```python
from build123d import *

# Parameters (mm, degrees)
F0_W          = 279.4
F0_H          = 279.4
F0_R          = 12.7
F1_DEPTH      = 76.2
F0_W_2        = 304.8
F0_H_2        = 304.8
F2_DEPTH      = 101.6
F2_DEPTH_BACK = 88.9
F3_R          = 50.8
F4_W          = 241.3
F4_H          = 241.3
F5_DEPTH      = 139.7
F6_DEPTH      = 101.6


with BuildPart() as f1:
    # F0 (on Top) → F1 (new body, symmetric)
    with BuildSketch(Plane.XY):
        Rectangle(F0_W, F0_H)
        Circle(F0_R, mode=Mode.SUBTRACT)
    extrude(amount=F1_DEPTH, both=True)

    # F0 (on Top) → F2 (join, two sides)
    with BuildSketch(Plane.XY) as f2_sk:
        Rectangle(F0_W_2, F0_H_2)
        Rectangle(F0_W, F0_H, mode=Mode.SUBTRACT)
    extrude(amount=F2_DEPTH)
    extrude(f2_sk.sketch, amount=-F2_DEPTH_BACK)

    # F3
    f3_edges = [f1.edges().sort_by_distance(p)[0] for p in [
        (152.4, -152.4, 6.35),
        (152.4, 152.4, 6.35),
        (-152.4, 152.4, 6.35),
        (-152.4, -152.4, 6.35),
        (-139.7, -139.7, 88.9),
        (-139.7, -139.7, -82.55),
        (-139.7, 139.7, 88.9),
        (-139.7, 139.7, -82.55),
        (139.7, 139.7, 88.9),
        (139.7, 139.7, -82.55),
        (139.7, -139.7, 88.9),
        (139.7, -139.7, -82.55),
    ]]
    fillet(f3_edges, radius=F3_R)

    # F4 (on face) → F5 (cut)
    with BuildSketch(Plane(origin=(0, 0, -76.2), x_dir=(1, 0, 0), z_dir=(0, 0, -1))):
        Rectangle(F4_W, F4_H)
    extrude(amount=-F5_DEPTH, mode=Mode.SUBTRACT)

    # F0 (on Top) → F6 (join)
    with BuildSketch(Plane.XY):
        Circle(F0_R)
    extrude(amount=F6_DEPTH)


solid = f1.part
```
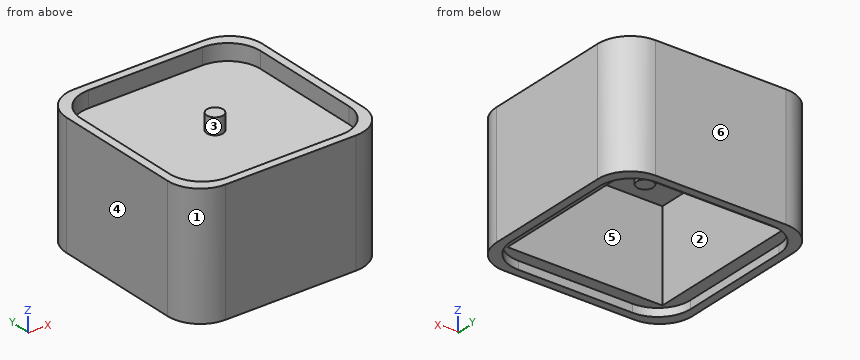
Source: CAD feature listing. Evaluate the final solid. Frame: model axes, mm. Face numbers are marked on the shaded views. A direction names the side the tool comes from. Coordinates: 2 decimals unless noted, no trailing zeros. Loops run counter-clockwise (first coordinate to the right, second up) from the corner with the lowest first, then second, coordinate; pieces in that order, holes last. Notation, with made-up numbers: M 34,86 L 41,86 A11 cw 41,92 Z; hole C 75,-32 d5. An arc over 180 degrees is marked long. Put each result on its own line as item: value. Start each with the question number.
1) Ray query, L1, parallel to Y at x = 52.5, z = -15; L2, parallel to X at y = 3.5, z = 45.5. Return the intervals inside material, ascending. Write a range as from..to.
2) Pull-direction query (X, two-part tool) for the marked faces 4, 5 and 6; classes: pulls with the +X half, pulls with the -X half, needs draft (parallel to the pull), parting line crosses it, or undercut.
3) Cut plane D-D on z = -47.5. Return the cut outline in (x, y).
4) Cut plane B-B on y = -23. Return the cut outline in (x, z).
5) Cut plane A-A on z = 80.5. Return the cut outline in (x, y), then the cut area to 3 significant figures.
6) Reachability of the marked faces 1, 2 and 3 from +Z, -Z, +X, -X, +Y, -Y: full face, straight path, thin tool, end or side. Return the list, or none.
7) Contact query for flat-ended pins moving along their axis: pin 1 Ø5 at (x, y) = (-39, -41.5) entering from +Z; pin 2 Ø4 at (x, y) = (-41, 41) entering from -Z; pin 3 Ø8 at (y, z) = (-115, -43.5) entering from -X. Output: stop coordinate, or through.
The answers:
1. L1: y = -152.4..-120.65, 120.65..152.4
1. L2: x = -152.4..-120.65, -12.21..12.21, 120.65..152.4
2. face 4: pulls with the -X half
2. face 5: undercut
2. face 6: needs draft
3. outline: M -152.4,-101.6 A50.8 ccw -101.6,-152.4 L 101.6,-152.4 A50.8 ccw 152.4,-101.6 L 152.4,101.6 A50.8 ccw 101.6,152.4 L -101.6,152.4 A50.8 ccw -152.4,101.6 Z; hole M -120.65,-120.65 L 120.65,-120.65 L 120.65,120.65 L -120.65,120.65 Z
4. outline: M -152.4,-88.9 L -139.7,-88.9 L -139.7,-76.2 L -120.65,-76.2 L -120.65,63.5 L 120.65,63.5 L 120.65,-76.2 L 139.7,-76.2 L 139.7,-88.9 L 152.4,-88.9 L 152.4,101.6 L 139.7,101.6 L 139.7,76.2 L -139.7,76.2 L -139.7,101.6 L -152.4,101.6 Z
5. outline: M -152.4,-101.6 A50.8 ccw -101.6,-152.4 L 101.6,-152.4 A50.8 ccw 152.4,-101.6 L 152.4,101.6 A50.8 ccw 101.6,152.4 L -101.6,152.4 A50.8 ccw -152.4,101.6 Z; C 0,0 d25.4; hole M -139.7,-88.9 A50.8 ccw -88.9,-139.7 L 88.9,-139.7 A50.8 ccw 139.7,-88.9 L 139.7,88.9 A50.8 ccw 88.9,139.7 L -88.9,139.7 A50.8 ccw -139.7,88.9 Z
5. area: 15,300 mm²
6. face 1: +Z, -Z, -X, -Y
6. face 2: -Z
6. face 3: +Z
7. pin 1: stops at z = 76.2
7. pin 2: stops at z = 63.5
7. pin 3: stops at x = -151.52
